For this review, take the finished solid that the model builds, in its own axes (mm). A direction names the side the tool comes from. Coordinates: 2 decimals unless noted, no trailing zeros. Write each loop counter-clockwise with the first axis right and the second up, starting at its lowest first coordinate (ties: lowest second). Pieces come first, ordered by that corner, then holes. Notation, with made-up numbers: (9, 42) -> (55, 42) arc R21 ccw to (55, 60) -> close; hole circle Ø11 at (-1.75, 21). An arc over 180 degrees is marked (long way). Put each result on its own line as item: value. Start each with the question number.
Item 1: The part is to be moulded in two halves that separate along X. For faces 1 (the flat face through (2, 0, 7)), 2 (the cylindrical face through (140, 0, 3)), 3 (the cylindrical face through (-132, 0, 4)), say which applies: +X half, -X half, draft (parallel to the pull), parting line (faces both ways), or undercut.
Item 2: Consider section A-A on y = 0. Give the boundary of the cut face in (x, z).
Item 3: Consider section C-C on z = 11.5. Give the boundary of the cut face in (x, y), and give its area (3 significant figures).
Item 4: Consider section D-D on y = -10. Give the boundary of the cut face in (x, z).
Item 5: To check wall thickness, follow L1, parallel to Y at x = -125, z = 4; L2, parallel to Z at x = -115, y = 0.5; L3, parallel to Y at x = -119, z = 6.75. State the ranges of each line that lie inside material, in increasing order.
Item 6: Insertion check: P1, Ø2, axis at x = -50.5, y = 0, coming from the +Z side; P2, Ø4, axis at y = 10, z = 2.5, coming from the +X side. Each pin has a flat end and moves straight along its axis. Give the tip position at first contact, or say it passes through.
Item 7: For faces 4 (the flat face through (2, -15, 3)), 5 (the cylindrical face through (118, 0, 10)), list the 3-axis set-ups (+Z, -Z, +X, -X, +Y, -Y) from which the entire face can be reached by the end or side of a thin tool; tool diameter is ignored.
Item 8: Consider section B-B on x = 89.5. Give the boundary of the cut face in (y, z).
```python
from build123d import *

# Parameters (mm, degrees)
BOSS_EXTRUDE1_DEPTH = 7
SKETCH2_R           = 7
BOSS_EXTRUDE2_DEPTH = 7
SKETCH3_R           = 7
CUT_EXTRUDE1_DEPTH  = 7


with BuildPart() as part:
    # Sketch1 → Boss-Extrude1 (new body)
    with BuildSketch(Plane.XY):
        with BuildLine():
            Line((-125, 15), (125, 15))
            ThreePointArc((125, 15), (140, 0), (125, -15))
            Line((125, -15), (-125, -15))
            ThreePointArc((-125, -15), (-140, 0), (-125, 15))
        make_face()
    extrude(amount=BOSS_EXTRUDE1_DEPTH)

    # Sketch2 → Boss-Extrude2 (add)
    with BuildSketch(Plane.XY.offset(7)):
        with Locations((125, 0)):
            Circle(SKETCH2_R)
    extrude(amount=BOSS_EXTRUDE2_DEPTH)

    # Sketch3 → Cut-Extrude1 (cut)
    with BuildSketch(Plane.XY.offset(7)):
        with Locations((-125, 0)):
            Circle(SKETCH3_R)
    extrude(amount=-CUT_EXTRUDE1_DEPTH, mode=Mode.SUBTRACT)


solid = part.part
```
Return value:
1. face 1: draft
1. face 2: +X half
1. face 3: undercut
2. outline: (-140, 0) -> (-132, 0) -> (-132, 7) -> (-140, 7) -> close; (-118, 0) -> (140, 0) -> (140, 7) -> (132, 7) -> (132, 14) -> (118, 14) -> (118, 7) -> (-118, 7) -> close
3. outline: circle Ø14 at (125, 0)
3. area: 154 mm^2
4. outline: (-136.18, 0) -> (136.18, 0) -> (136.18, 7) -> (-136.18, 7) -> close
5. L1: -15 to -7, 7 to 15
5. L2: 0 to 7
5. L3: -15 to -3.61, 3.61 to 15
6. P1: z = 7
6. P2: x = 137.69
7. face 4: +Z, -Z, +X, -X, -Y
7. face 5: +Z
8. outline: (-15, 0) -> (15, 0) -> (15, 7) -> (-15, 7) -> close
